Part model, mm, in its own coordinate system. Face numbers are marked on the shaded views. A direction names the side the tool comes from. Round coordinates to 2 decimals unless told otherwise and drop trailing zeros. Loops run counter-clockwise (first coordinate to the right, second up) from the corner with the lowest first, then second, coordinate; pieces in that order, holes last.
from build123d import *

# Parameters (mm, degrees)
F0_W           = 20
F0_H           = 20
F1_DEPTH       = 2
F0_W_2         = 5
F2_DEPTH       = 4
F3_W           = 16.8
F3_H           = 16.8
F4_DEPTH       = 20
F5_SIZE        = 1
F6_D           = 5
F6_CSINK_D     = 10
F6_CSINK_ANGLE = 90


with BuildPart() as f1:
    # F0 (on Top) → F1 (new body)
    with BuildSketch(Plane.XY):
        with Locations((15, 10)):
            Rectangle(F0_W, F0_H)
    extrude(amount=F1_DEPTH)

    # F0 (on Top) → F2 (join)
    with BuildSketch(Plane.XY):
        with Locations((2.5, 10)):
            Rectangle(F0_W_2, F0_H)
        with BuildLine():
            ThreePointArc((0, 20), (-10, 10), (0, 0))
            Line((0, 0), (0, 20))
        make_face()
        with Locations((15, 10)):
            Rectangle(F0_W, F0_H)
        with Locations((27.5, 10)):
            Rectangle(F0_W_2, F0_H)
        with BuildLine():
            Line((30, 20), (30, 0))
            ThreePointArc((30, 0), (40, 10), (30, 20))
        make_face()
    extrude(amount=-F2_DEPTH)

    # F3 (on face) → F4 (join)
    with BuildSketch(Plane.XY.offset(2)):
        with Locations((15, 10)):
            Rectangle(F3_W, F3_H)
    extrude(amount=F4_DEPTH)

    # F5
    f5_edges = [f1.edges().sort_by_distance(p)[0] for p in [
        (23.4, 18.4, 12),
        (6.6, 18.4, 12),
        (15, 18.4, 22),
        (6.6, 10, 22),
        (23.4, 10, 22),
        (15, 1.6, 22),
        (23.4, 1.6, 12),
        (6.6, 1.6, 12),
    ]]
    chamfer(f5_edges, length=F5_SIZE)

    # F6 (through all)
    with Locations(Plane.XY):
        with Locations((-4, 10), (34, 10)):
            CounterSinkHole(F6_D / 2, F6_CSINK_D / 2, counter_sink_angle=F6_CSINK_ANGLE)


solid = f1.part
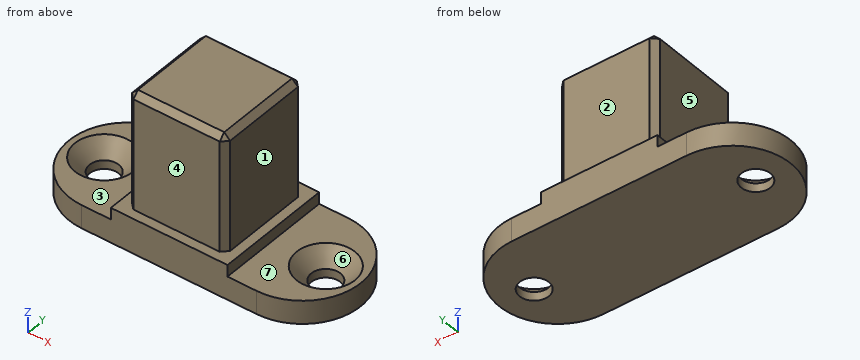
1) Slice it at D-D, the plane y = 3.75. Give the cut face in (x, z).
Values:
outline: (-7.81, -4) - (37.81, -4) - (37.81, 0) - (25, 0) - (25, 2) - (23.4, 2) - (23.4, 21) - (22.4, 22) - (7.6, 22) - (6.6, 21) - (6.6, 2) - (5, 2) - (5, 0) - (-7.81, 0) - close
2) Tool access for the marked faces 1, 2, 3 and 4: list every direction of +Z, -Z, +X, -X, +Y, -Y with a clear straight run to the whole face (end or side of a thin tool).
Values:
face 1: +Z, +X, +Y, -Y
face 2: +Z, +X, -X, +Y
face 3: +Z, -X, +Y, -Y
face 4: +Z, +X, -X, -Y
3) Slice it at B-B, the plane x = -4. Give the cut face in (y, z), then the cut area to 3 significant figures.
Values:
outline: (0.83, -4) - (7.5, -4) - (7.5, -2.5) - (5, 0) - (0.83, 0) - close; (12.5, -4) - (19.17, -4) - (19.17, 0) - (15, 0) - (12.5, -2.5) - close
area: 47.1 mm2
4) Slice it at A-A, the plane y = 10. Give the cut face in (x, z).
Values:
outline: (-10, -4) - (-6.5, -4) - (-6.5, -2.5) - (-9, 0) - (-10, 0) - close; (-1.5, -4) - (31.5, -4) - (31.5, -2.5) - (29, 0) - (25, 0) - (25, 2) - (23.4, 2) - (23.4, 21) - (22.4, 22) - (7.6, 22) - (6.6, 21) - (6.6, 2) - (5, 2) - (5, 0) - (1, 0) - (-1.5, -2.5) - close; (36.5, -4) - (40, -4) - (40, 0) - (39, 0) - (36.5, -2.5) - close
5) Slice it at C-C, the plane z = 2.5. Give the cut face in (x, y).
Values:
outline: (6.6, 2.6) - (7.6, 1.6) - (22.4, 1.6) - (23.4, 2.6) - (23.4, 17.4) - (22.4, 18.4) - (7.6, 18.4) - (6.6, 17.4) - close
6) Wall check: line 1 along X through (y, z) = (10, -3.25); line 2 along X through (y, z) = (2.75, 3.75); line 3 along Y through (x, z) = (13.5, 9). Give the ranges that are in metal, low to high.
Values:
line 1: x = -10 to -6.5, -1.5 to 31.5, 36.5 to 40
line 2: x = 6.6 to 23.4
line 3: y = 1.6 to 18.4
7) Mould opens along X. For the marked faces 5, 6 and 7 say: released by +X, released by -X, zero draft, split by the parting line, or undercut.
Values:
face 5: released by -X
face 6: undercut
face 7: zero draft
8) Drop flat-ended pins along their axis: pin 1 Ø8 at (y, z) = (2.5, -1) entering from +X; pin 2 Ø10 at (x, y) = (35, 6) entering from +Z; pin 3 Ø0.6 at (y, z) = (5.5, 1.5) entering from +X. Give the stop position or say it passes through.
Values:
pin 1: stops at x = 39.37
pin 2: stops at z = 0
pin 3: stops at x = 25
